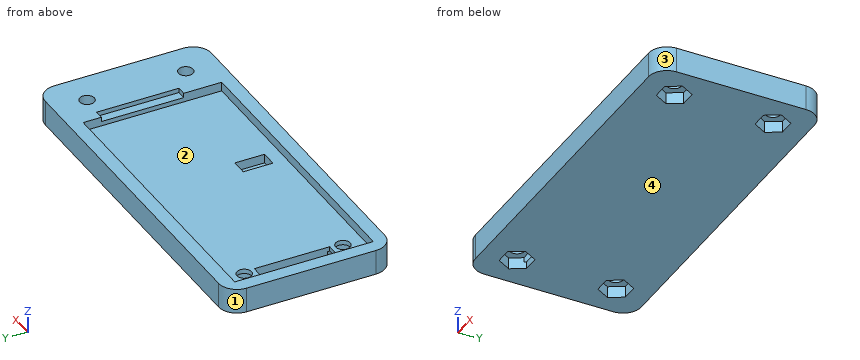
from build123d import *

# Parameters (mm, degrees)
F0_W      = 80
F0_H      = 36.3
F1_DEPTH  = 5.5
F2_R      = 4
F3_W      = 63
F3_H      = 30.3
F4_DEPTH  = 2
F5_W      = 5
F5_H      = 16.5
F5_W_2    = 3.5
F5_H_2    = 6.5
F6_DEPTH  = 4
F7_W      = 2
F7_H      = 18
F8_DEPTH  = 1
F9_R      = 1.6
F10_DEPTH = 5.501
F12_DEPTH = 2.5


with BuildPart() as f1:
    # F0 (on Top) → F1 (new body)
    with BuildSketch(Plane.XY):
        with Locations((37, 15.15)):
            Rectangle(F0_W, F0_H)
    extrude(amount=F1_DEPTH)

    # F2
    f2_edges = [f1.edges().sort_by_distance(p)[0] for p in [
        (-3, -3, 2.75),
        (77, -3, 2.75),
        (77, 33.3, 2.75),
        (-3, 33.3, 2.75),
    ]]
    fillet(f2_edges, radius=F2_R)

    # F3 (on face) → F4 (cut)
    with BuildSketch(Plane.XY.offset(5.5)):
        with Locations((31.5, 15.15)):
            Rectangle(F3_W, F3_H)
    extrude(amount=-F4_DEPTH, mode=Mode.SUBTRACT)

    # F5 (on face) → F6 (cut)
    with BuildSketch(Plane.XY.offset(5.5)):
        with Locations((2.5, 15.15)):
            Rectangle(F5_W, F5_H)
        with Locations((37.75, 6.25)):
            Rectangle(F5_W_2, F5_H_2)
    extrude(amount=-F6_DEPTH, mode=Mode.SUBTRACT)

    # F7 (on face) → F8 (cut)
    with BuildSketch(Plane.XY.offset(5.5)):
        with Locations((64, 17.3)):
            Rectangle(F7_W, F7_H)
    extrude(amount=-F8_DEPTH, mode=Mode.SUBTRACT)

    # F9 (on face) → F10 (cut, through all)
    with BuildSketch(Plane.XY.offset(5.5)):
        with Locations((4.35, 4.35)):
            Circle(F9_R)
        with Locations((4.35, 25.95)):
            Circle(F9_R)
        with Locations((69.65, 25.95)):
            Circle(F9_R)
        with Locations((69.65, 4.35)):
            Circle(F9_R)
    extrude(amount=-F10_DEPTH, mode=Mode.SUBTRACT)

    # F11 (on face) → F12 (cut)
    with BuildSketch(Plane(origin=(0, 0, 0), x_dir=(1, 0, 0), z_dir=(0, 0, -1))):
        Polygon((67.917949, -28.95), (71.382051, -28.95), (73.114102, -25.95), (71.382051, -22.95), (67.917949, -22.95), (66.185898, -25.95), align=None)
        Polygon((73.114102, -4.35), (71.382051, -1.35), (67.917949, -1.35), (66.185898, -4.35), (67.917949, -7.35), (71.382051, -7.35), align=None)
        Polygon((7.814102, -25.95), (6.082051, -22.95), (2.617949, -22.95), (0.885898, -25.95), (2.617949, -28.95), (6.082051, -28.95), align=None)
        Polygon((7.814102, -4.35), (6.082051, -1.35), (2.617949, -1.35), (0.885898, -4.35), (2.617949, -7.35), (6.082051, -7.35), align=None)
    extrude(amount=-F12_DEPTH, mode=Mode.SUBTRACT)


solid = f1.part
Check sheet for the modelled part. Datum: model origin and axes. Units: mm. Face numbers are marked on the shaded views. Coordinates: 2 decimals unless noted, no trailing zeros. Loops run counter-clockwise (first coordinate to the right, second up) from the corner with the lowest first, then second, coordinate; pieces in that order, holes last. Notation, with made-up numbers: (7.25, -17.75) -> (48.25, -17.75) arc R37 cw to (48.25, 21.25) -> close; hole circle Ø2 at (82.25, 11.25). An arc over 180 degrees is marked (long way). Write item = value, one per line. Start each with the question number.
1. Material ranges on line 1 (Y direction, x = 69.65, z = 4.75); line 2 (X direction, y = 13, z = 4); line 3 (Y direction, x = 31, z = 3.75), recorded low to high.
2. Depth check by flat-ended pin: P1, Ø1, axis at x = 64, y = 18, coming from the +Z side. Enter the tip coordinate at first touch or a pass-through.
3. Section check A-A on x = 69.65. Record the cut outline in (y, z), then the cut area to 3 significant figures.
4. Draft check along X on the marked faces 1, 2, 3 and 4. Enter one of: released by +X, released by -X, zero draft, split by the parting line, or undercut.
5. Section check B-B on y = 11. Record the cut outline in (x, z).
6. Section check C-C on x = 55.5. Record the cut outline in (y, z), then the cut area to 3 significant figures.
Responses:
q1.line_1 = -3 to 2.75, 5.95 to 24.35, 27.55 to 33.3
q1.line_2 = -3 to 0, 63 to 77
q1.line_3 = -3 to 0, 30.3 to 33.3
q2.P1 = 4.5
q3.outline = (-3, 0) -> (1.35, 0) -> (1.35, 2.5) -> (2.75, 2.5) -> (2.75, 5.5) -> (-3, 5.5) -> close; (5.95, 2.5) -> (7.35, 2.5) -> (7.35, 0) -> (22.95, 0) -> (22.95, 2.5) -> (24.35, 2.5) -> (24.35, 5.5) -> (5.95, 5.5) -> close; (27.55, 2.5) -> (28.95, 2.5) -> (28.95, 0) -> (33.3, 0) -> (33.3, 5.5) -> (27.55, 5.5) -> close
q3.area = 150 mm2
q4.face_1 = released by -X
q4.face_2 = undercut
q4.face_3 = released by +X
q4.face_4 = zero draft
q5.outline = (-3, 0) -> (77, 0) -> (77, 5.5) -> (65, 5.5) -> (65, 4.5) -> (63, 4.5) -> (63, 3.5) -> (5, 3.5) -> (5, 1.5) -> (0, 1.5) -> (0, 5.5) -> (-3, 5.5) -> close
q6.outline = (-3, 0) -> (33.3, 0) -> (33.3, 5.5) -> (30.3, 5.5) -> (30.3, 3.5) -> (0, 3.5) -> (0, 5.5) -> (-3, 5.5) -> close
q6.area = 139 mm2
